Geometry check sheet. Reference: the model listing, model coordinates, mm. A direction names the side the tool comes from. Round coordinates to 2 decimals unless told otherwise and drop trailing zeros. Loops run counter-clockwise (first coordinate to the right, second up) from the corner with the lowest first, then second, coordinate; pieces in that order, holes last. Notation, with made-up numbers: M 8.25,59.5 L 55.25,59.5 A27 cw 55.25,89.5 Z; hole C -23,-25.5 d11. An arc over 180 degrees is marked long. Use one line per item in the form item = value. Start each with the question number.
1. Cross-section at A-A (y = 0). Record the boundary of the cut face in (x, z), then the cut area to 3 significant figures.
2. Go/stop test with flat-tipped pins: pin 1 (12 mm diameter, centred on x = 35, y = -6.5, fed in from -Z); pin 2 (3 mm diameter, centred on x = 56.5, y = -51, fed in from -Z); pin 3 (4 mm diameter, centred on x = 11, y = -35, fed in from -Z). Record where each tip stops, or that it passes through.
3. Material ranges on line 1 (X direction, y = -53, z = 167.5); line 2 (Y direction, x = -1.5, z = -22); line 3 (Z direction, x = 41.5, y = -42), recorded low to high.
4. Cross-section at B-B (x = 30). Record the boundary of the cut face in (y, z), then the cut area to 3 significant figures.
5. Cross-section at C-C (z = 190). Record the boundary of the cut face in (x, y).
6. Set-up check for faces 1 (the cylindrical face through (75.07, 7.509, -23.846)), 2 (the cylindrical face through (-4.93, 7.509, -23.846)), 3 (the flat face through (-10, 0, 0)): record each of +Z, -Z, +X, -X, +Y, -Y from which the full face is reachable in a straight line by a thin tool's end or side.
```python
from build123d import *

# Parameters (mm, degrees)
SKETCH3_R           = 70
BOSS_EXTRUDE1_DEPTH = 70
SKETCH4_R           = 25
BOSS_EXTRUDE2_DEPTH = 10
BOSS_EXTRUDE3_START = 10
SKETCH6_R           = 25
BOSS_EXTRUDE3_DEPTH = 10
SKETCH7_W           = 70
SKETCH7_H           = 400
BOSS_EXTRUDE4_DEPTH = 140
BOSS_EXTRUDE5_START = -70
BOSS_EXTRUDE5_DEPTH = 70
BOSS_EXTRUDE6_DEPTH = 70


with BuildPart() as part:
    # Sketch3 → Boss-Extrude1 (new body)
    with BuildSketch(Plane(origin=(0, 0, 0), x_dir=(0, 0, -1), z_dir=(1, 0, 0))):
        Circle(SKETCH3_R)
    extrude(amount=BOSS_EXTRUDE1_DEPTH)

    # Sketch4 → Boss-Extrude2 (add)
    with BuildSketch(Plane(origin=(0, 0, 0), x_dir=(0, 0, -1), z_dir=(1, 0, 0))):
        Circle(SKETCH4_R)
    extrude(amount=-BOSS_EXTRUDE2_DEPTH)

    # Sketch6 → Boss-Extrude3 (add)
    with BuildSketch(Plane(origin=(70, 0, 0), x_dir=(0, 0, -1), z_dir=(1, 0, 0)).offset(BOSS_EXTRUDE3_START)):
        Circle(SKETCH6_R)
    extrude(amount=-BOSS_EXTRUDE3_DEPTH)



with BuildPart() as body_2:
    # Sketch7 → Boss-Extrude4 (new body)
    with BuildSketch(Plane(origin=(0, 70, 0), x_dir=(1, 0, 0), z_dir=(0, 1, 0))):
        with Locations((35, -270)):
            Rectangle(SKETCH7_W, SKETCH7_H)
    extrude(amount=-BOSS_EXTRUDE4_DEPTH)


with BuildPart() as part_1:
    add(part.part)

    add(body_2.part)  # Boss-Extrude5 merges body 2
    # Sketch8 → Boss-Extrude5 (add)
    with BuildSketch(Plane(origin=(70, 0, 0), x_dir=(0, 0, -1), z_dir=(1, 0, 0)).offset(BOSS_EXTRUDE5_START)):
        with BuildLine():
            ThreePointArc((-70, -2.7e-08), (-49.497474693, 49.497474674), (0, 70))
            Line((0, 70), (-70, 70))
            Line((-70, 70), (-70, -2.7e-08))
        make_face()
        with BuildLine():
            ThreePointArc((0, -70), (-49.497474674, -49.497474693), (-70, -2.7e-08))
            Line((-70, -2.7e-08), (-70, -70))
            Line((-70, -70), (0, -70))
        make_face()
    extrude(amount=BOSS_EXTRUDE5_DEPTH)

    # Sketch9 → Boss-Extrude6 (add)
    with BuildSketch(Plane(origin=(0, 0, 0), x_dir=(0, 0, -1), z_dir=(1, 0, 0))):
        with BuildLine():
            Line((-470, 70), (-470, -70))
            ThreePointArc((-470, -70), (-540, 0), (-470, 70))
        make_face()
    extrude(amount=BOSS_EXTRUDE6_DEPTH)


solid = part_1.part
```
Reported:
q1.outline = M -10,-25 L 0,-25 L 0,-70 L 70,-70 L 70,-25 L 80,-25 L 80,25 L 70,25 L 70,540 L 0,540 L 0,25 L -10,25 Z
q1.area = 43,700 mm²
q2.pin_1 = -70
q2.pin_2 = -49.49
q2.pin_3 = -61.73
q3.line_1 = 0 to 70
q3.line_2 = -11.87 to 11.87
q3.line_3 = -56 to 526
q4.outline = M -70,0 A70 ccw 70,0 L 70,470 A70 ccw -70,470 Z
q4.area = 81,200 mm²
q5.outline = M 0,-70 L 70,-70 L 70,70 L 0,70 Z
q6.face_1 = +X
q6.face_2 = -X
q6.face_3 = +Z, -Z, -X, +Y, -Y
